Can you work these out from the model? Positions are in its coordinate system, mm. A direction names the side the tool comes from. Coordinates: 2 decimals unless noted, no trailing zeros. Write each loop counter-clockwise with the first axis right and the second up, starting at its lowest first coordinate (ties: lowest second). Pieces come first, ordered by that corner, then holes. Notation, with made-up numbers: (28.5, 11.25) -> (38.5, 11.25) arc R14 cw to (38.5, 32.25) -> close; hole circle Ø9 at (-29, 56.5). An arc over 180 degrees is marked (long way). Use one line per item in the form item = value.
```python
from build123d import *

# Parameters (mm, degrees)
F1_DEPTH = 7.366


with BuildPart() as f1:
    # F0 (on Front) → F1 (new body)
    with BuildSketch(Plane.XZ):
        Polygon((4.967066, 29.668139), (-3.087636, 29.668139), (-7.114984, 29.668139), (-7.114984, 26.446259), (-10.605352, 26.446259), (-10.605352, 23.22438), (-14.095721, 23.22438), (-14.095721, 17.049111), (-19.197032, 17.049111), (-18.66005, 7.114983), (-24.029849, 7.114983), (-24.029849, 4.698574), (-25.909279, 4.698574), (-25.909279, -2.013674), (-24.029849, -2.013674), (-24.029849, -20.002501), (-25.909279, -20.002501), (-25.909279, -25.640789), (-28.325688, -25.640789), (-28.325688, -27.788708), (-28.325688, -32.890018), (-16.24364, -32.890018), (-16.24364, -25.640789), (-7.114984, -25.640789), (-7.114984, -27.788708), (-10.605352, -27.788708), (-10.605352, -32.890018), (8.725923, -32.890018), (8.725923, -27.788708), (5.504044, -27.788708), (5.504044, -25.640789), (15.975151, -25.640789), (15.975151, -32.890018), (26.177768, -32.890018), (26.177768, -25.640789), (24.029847, -25.640789), (24.029847, -20.002501), (20.80797, -20.002501), (20.80797, -2.013674), (24.029847, -2.013674), (24.029847, 4.698574), (20.80797, 4.698574), (20.80797, 7.114983), (15.975151, 7.114983), (15.975151, 17.317601), (13.827233, 17.317601), (13.827233, 21.881929), (11.410821, 21.881929), (11.410821, 24.298338), (8.725923, 24.298338), (8.725923, 26.714748), (4.967066, 26.714748), align=None)
    extrude(amount=F1_DEPTH)


solid = f1.part
```
Q1. If I drill on line 1 (X direction, y = -3.75, z = -28); line 2 (Z direction, x = 22, y = -3); line 3 (Z direction, x = -23, y = -2.25), over which ranges is the centre line in solid material (lowest first)? Write a range as from..to.
Return value:
line_1 = -28.33..-16.24, -10.61..8.73, 15.98..26.18
line_2 = -32.89..-20, -2.01..4.7
line_3 = -32.89..7.11
Q2. For faces 5 (the flat face through (-9, -4, -27.789)), 6 (the flat face through (10, -4, 24.298)), 7 (the flat face through (-25.909, -4, 1)), 8 (the flat face through (-10.605, -4, -30)), which set-ups out of +Z, -Z, +X, -X, +Y, -Y let a thin tool reach every point of the face, with its end or its side?
Return value:
face_5 = +Y, -Y
face_6 = +Z, +X, +Y, -Y
face_7 = +Z, -X, +Y, -Y
face_8 = -Z, +Y, -Y
Q3. Suppose I cut it at A-A (x = 7). Write out the boundary of the cut face in (y, z), then the cut area to 3 significant figures.
Return value:
outline = (-7.37, -32.89) -> (0, -32.89) -> (0, -27.79) -> (-7.37, -27.79) -> close; (-7.37, -25.64) -> (0, -25.64) -> (0, 26.71) -> (-7.37, 26.71) -> close
area = 423 mm2
Q4. Suppose I cut it at C-C (x = 21.5). Write out the boundary of the cut face in (y, z), then the cut area to 3 significant figures.
Return value:
outline = (-7.37, -32.89) -> (0, -32.89) -> (0, -20) -> (-7.37, -20) -> close; (-7.37, -2.01) -> (0, -2.01) -> (0, 4.7) -> (-7.37, 4.7) -> close
area = 144 mm2
Q5. Thinking about a two-plate mould opening in Z: for faces 1 (the flat face through (-25, -4, -2.014)), 2 (the flat face through (-10.605, -4, 25)), 3 (the flat face through (-24.03, -4, -11)), 4 (the flat face through (-25, -4, 4.699)), which applies, released by +Z, released by -Z, zero draft, split by the parting line, or undercut?
Return value:
face_1 = undercut
face_2 = zero draft
face_3 = undercut
face_4 = released by +Z
Q6. Suppose I cut it at D-D (x = 13). Write out the boundary of the cut face in (y, z).
Return value:
outline = (-7.37, -25.64) -> (0, -25.64) -> (0, 21.88) -> (-7.37, 21.88) -> close
Q7. Will these pins go through, and if not, where does the flat tip stop? pin 1 (2.5 mm diameter, centred on x = 8, y = -5, fed in from +Z); pin 2 (0.9 mm diameter, centred on x = -25.5, y = -3.5, fed in from +Z); pin 3 (1.1 mm diameter, centred on x = 25, y = -3.5, fed in from +Z).
Return value:
pin_1 = 26.71
pin_2 = 4.7
pin_3 = -25.64
Q8. Suppose I cut it at B-B (z = -27). Write out the boundary of the cut face in (x, y), then the cut area to 3 significant figures.
Return value:
outline = (-28.33, -7.37) -> (-16.24, -7.37) -> (-16.24, 0) -> (-28.33, 0) -> close; (-7.11, -7.37) -> (5.5, -7.37) -> (5.5, 0) -> (-7.11, 0) -> close; (15.98, -7.37) -> (26.18, -7.37) -> (26.18, 0) -> (15.98, 0) -> close
area = 257 mm2
